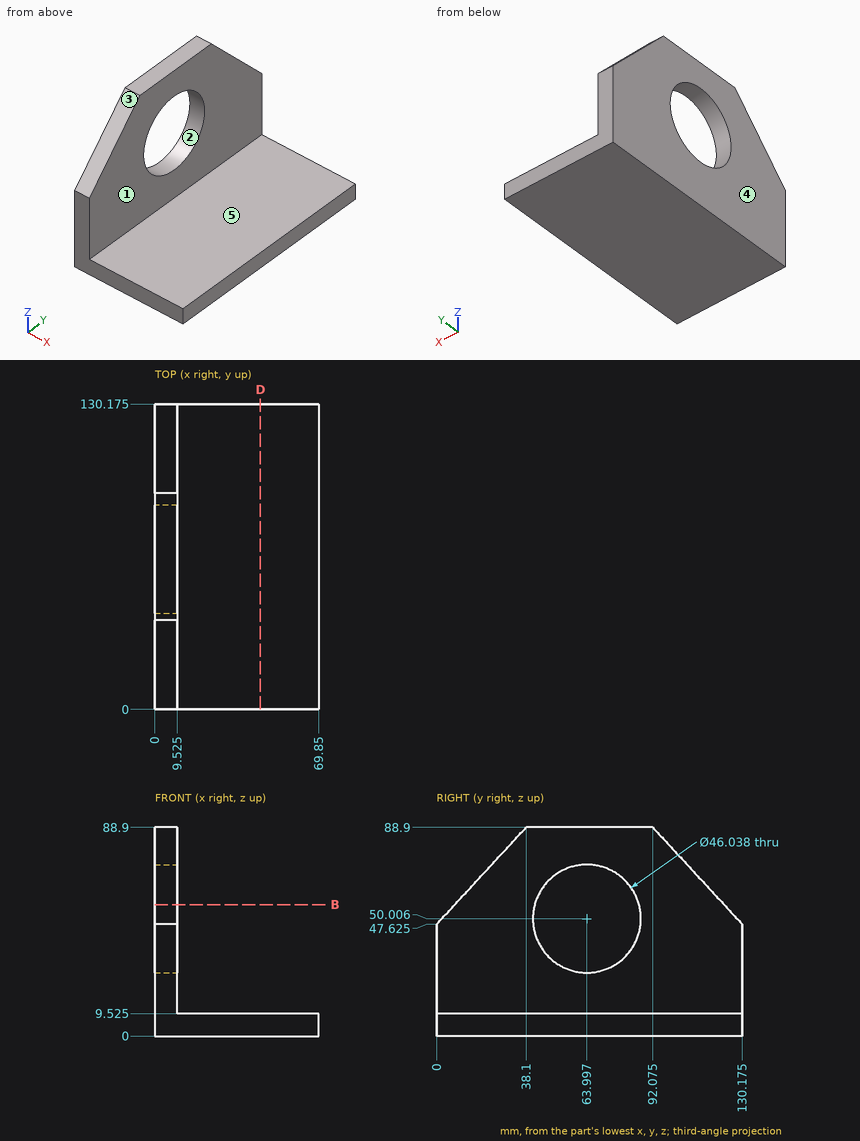
Study the drawing (mm; zero at the part's minimum x, y, z) and answer. A direction names the side the tool comes from. Coordinates: 2 decimals unless noted, no trailing zeros. Write each loop counter-clockwise with the first axis right and the second up, starting at its lowest first coordinate (ties: lowest second). Pieces come first, ordered by that corner, then holes.
Q1. Find the intervals of material crossed by line 1 (Z direction, x = 30.5, y = 37) (1 decimal), in increasing order.
Q2. Determine the mould class of the marked faces 1, 2 and 3 for opening direction Y: released by +Y, released by -Y, zero draft, split by the parting line, or undercut.
Q3. A cutting plane is placed at B-B, the plane z = 56. Give the vertices of the cut face in (x, y) (1 decimal).
Q4. A cutting plane is placed at D-D, the plane x = 45. Give the vertices of the cut face in (y, z) (1 decimal), then the cut area to 3 significant figures.
Q5. Each of these flat-tipped pins is pushed along its axis until it touches: pin 1 Ø5 at (x, y) = (52, 63.5) entering from +Z (1 decimal); pin 2 Ø12 at (y, z) = (90, 61) entering from +X (1 decimal). Where does it stop, or does it pass through?
Q6. Which of the six approach directions +Z, -Z, +X, -X, +Y, -Y give full straight-line access (tool end or side, diameter ignored) to the marked faces 4 and 5?
Findings below:
1. line 1: z = 0 to 9.5
2. face 1: zero draft
2. face 2: undercut
2. face 3: released by -Y
3. outline: (0, 7.7) - (9.5, 7.7) - (9.5, 41.8) - (0, 41.8) - close; (0, 86.2) - (9.5, 86.2) - (9.5, 122.4) - (0, 122.4) - close
4. outline: (0, 0) - (130.2, 0) - (130.2, 9.5) - (0, 9.5) - close
4. area: 1,240 mm2
5. pin 1: stops at z = 9.5
5. pin 2: stops at x = 9.5
6. face 4: +Z, -Z, -X, +Y, -Y
6. face 5: +Z, +X, +Y, -Y
